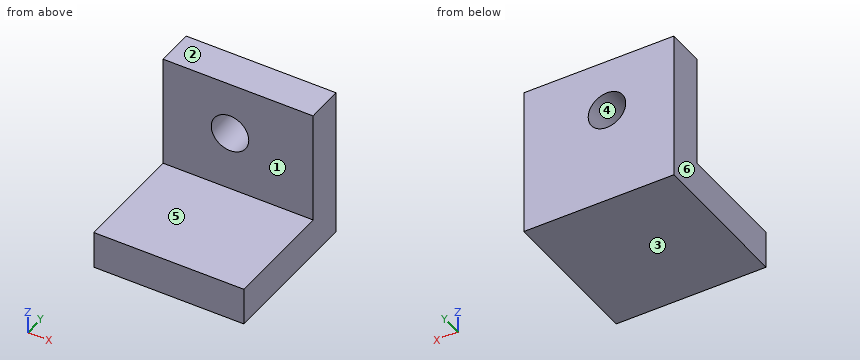
```python
from build123d import *

# Parameters (mm, degrees)
F0_W     = 50.8
F0_H     = 38.1
F1_DEPTH = 12.7
F0_H_2   = 12.7
F2_DEPTH = 50.8
F3_R     = 6.35
F4_DEPTH = 12.7


with BuildPart() as f1:
    # F0 (on Top) → F1 (new body)
    with BuildSketch(Plane.XY):
        with Locations((-30.416981, -6.624007)):
            Rectangle(F0_W, F0_H)
    extrude(amount=F1_DEPTH)

    # F0 (on Top) → F2 (join)
    with BuildSketch(Plane.XY):
        with Locations((-30.416981, 18.775993)):
            Rectangle(F0_W, F0_H_2)
    extrude(amount=F2_DEPTH)

    # F3 (on face) → F4 (cut)
    with BuildSketch(Plane.XZ.offset(-12.425993)):
        with Locations((-33.133555, 32.930352)):
            Circle(F3_R)
    extrude(amount=-F4_DEPTH, mode=Mode.SUBTRACT)


solid = f1.part
```
CAD build for the part. Positions are in the model's coordinates, mm. Face numbers are marked on the shaded views. A direction names the side the tool comes from. Give positions to 0.01 mm unless a question says otherwise; leave off trailing zeros. Write each loop counter-clockwise with the first axis right and the second up, starting at its lowest first coordinate (ties: lowest second). Pieces come first, ordered by that corner, then holes. Notation, with made-up numbers: (-27.5, -18) -> (1.5, -18) arc R33 cw to (1.5, 18) -> close; hole circle Ø11 at (-6, 68.25). An arc over 180 degrees is marked (long way). Write each question's results on one line, items separated by ' | '.
1. Two-plate mould, pull along Z, no slides. Class the marked faces 1, 2, 3 and 4: pulls with the +Z half, pulls with the -Z half, needs draft (parallel to the pull), parting line crosses it, or undercut.
Geometry check:
face 1: needs draft | face 2: pulls with the +Z half | face 3: pulls with the -Z half | face 4: undercut
2. Cut at B-B, the plane z = 34. Write the cut outline in (x, y), then the cut area to 3 significant figures.
Geometry check:
outline: (-55.82, 12.43) -> (-39.39, 12.43) -> (-39.39, 25.13) -> (-55.82, 25.13) -> close; (-26.87, 12.43) -> (-5.02, 12.43) -> (-5.02, 25.13) -> (-26.87, 25.13) -> close | area: 486 mm²
3. Cut at C-C, the plane y = 21. Write the cut outline in (x, z), then the cut area to 3 significant figures.
Geometry check:
outline: (-55.82, 0) -> (-5.02, 0) -> (-5.02, 50.8) -> (-55.82, 50.8) -> close; hole circle Ø12.7 at (-33.13, 32.93) | area: 2,450 mm²
4. Cut at A-A, the plane x = -30.5. Write the cut outline in (y, z).
Geometry check:
outline: (-25.67, 0) -> (25.13, 0) -> (25.13, 27.15) -> (12.43, 27.15) -> (12.43, 12.7) -> (-25.67, 12.7) -> close; (12.43, 38.71) -> (25.13, 38.71) -> (25.13, 50.8) -> (12.43, 50.8) -> close
5. Which spindle directions (+Z, -Z, +X, -X, +Y, -Y) get a long thin tool onto all of the face, cutting with end or side? Do the marked faces 5 and 6. Say none if no direction does.
Geometry check:
face 5: +Z, +X, -X, -Y | face 6: +Z, -Z, -X, +Y, -Y
6. Wall check: probe 1 along Z at (x, y) = (-38.5, -5); probe 2 along Y at (x, z) = (-52, 31); probe 3 along X at (y, z) = (18, 28.5). Give the ranges that are in metal, low to high. Write a range as [from, to].
Geometry check:
probe 1: [0, 12.7] | probe 2: [12.43, 25.13] | probe 3: [-55.82, -37.68], [-28.58, -5.02]
7. Drop flat-ended pins along their axis: P1, Ø10, axis at x = -33.13, z = 32.93, coming from the +Y side; P2, Ø1.5, axis at x = -49.5, z = 32, coming from the -Y side; P3, Ø5, axis at x = -40, y = 7.5, coming from the +Z side. Give the stop position or say it passes through.
Geometry check:
P1: through | P2: y = 12.43 | P3: z = 12.7
8. Cut at D-D, the plane x = -41.5. Write the cut outline in (y, z).
Geometry check:
outline: (-25.67, 0) -> (25.13, 0) -> (25.13, 50.8) -> (12.43, 50.8) -> (12.43, 12.7) -> (-25.67, 12.7) -> close
